Could you check a few things on this model? Use its own coordinates, in mm. Face numbers are marked on the shaded views. A direction names the side the tool comes from. Round coordinates to 2 decimals unless told otherwise and drop trailing zeros. Loops run counter-clockwise (first coordinate to the right, second up) from the corner with the lowest first, then second, coordinate; pieces in that order, holes last. Notation, with made-up numbers: M 34.25,-21 L 38.25,-21 A24 cw 38.25,2 Z; hole C -31.5,-25.5 d3. An arc over 180 degrees is marked long. Answer in a Markdown table with one row per item.
```python
from build123d import *

# Parameters (mm, degrees)
SKETCH018_R     = 1.75
PAD009_DEPTH    = 20
SKETCH019_W     = 27.500439
SKETCH019_H     = 11.45
SKETCH019_R     = 1.75
PAD010_DEPTH    = 4
SKETCH020_R     = 2.75
POCKET009_DEPTH = 8


with BuildPart() as part:
    # Sketch018 (on Face27 of Binder005) → Pad009 (new body)
    with BuildSketch(Plane.XZ.offset(-32.95)):
        Polygon((-0.000439, 13.05), (27.5, 13.05), (27.5, 1.6), (20.338297, 1.6), (20.338297, 3.6), (5.278297, 3.6), (5.278297, 1.6), (-0.000439, 1.6), align=None)
        with Locations((5.24978, 9.3)):
            Circle(SKETCH018_R, mode=Mode.SUBTRACT)
        with Locations((22.24978, 9.3)):
            Circle(SKETCH018_R, mode=Mode.SUBTRACT)
    extrude(amount=PAD009_DEPTH)

    # Sketch019 (on Face12 of Pad009) → Pad010 (join)
    with BuildSketch(Plane.XZ.offset(-12.95)):
        with Locations((13.74978, 7.325)):
            Rectangle(SKETCH019_W, SKETCH019_H)
        with Locations((5.24978, 9.3)):
            Circle(SKETCH019_R, mode=Mode.SUBTRACT)
        with Locations((22.24978, 9.3)):
            Circle(SKETCH019_R, mode=Mode.SUBTRACT)
    extrude(amount=PAD010_DEPTH)

    # Sketch020 (on Face1 of Pad010) → Pocket009 (cut)
    with BuildSketch(Plane.XZ.offset(-8.95)):
        with Locations((22.24978, 9.3)):
            Circle(SKETCH020_R)
        with Locations((5.24978, 9.3)):
            Circle(SKETCH020_R)
    extrude(amount=-POCKET009_DEPTH, mode=Mode.SUBTRACT)


solid = part.part
```
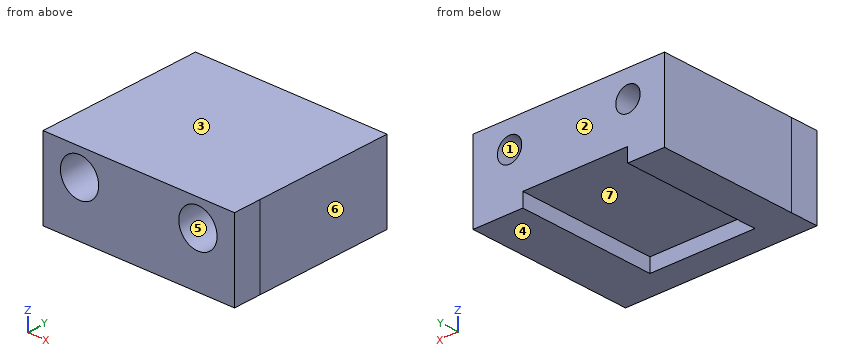
1) I want a section at C-C, the plane x = 19. Please give me the cut outline in (y, z), plus the area to 3 significant figures.
Computed:
| item | result |
|---|---|
| outline | M 8.95,1.6 L 12.95,1.6 L 12.95,3.6 L 32.95,3.6 L 32.95,13.05 L 8.95,13.05 Z |
| area | 235 mm² |
2) I want a section at B-B, the plane z = 9.3. Please give me the cut outline in (x, y).
Computed:
| item | result |
|---|---|
| outline | M 0,8.95 L 2.5,8.95 L 2.5,16.95 L 3.5,16.95 L 3.5,32.95 L 0,32.95 Z; M 7,16.95 L 8,16.95 L 8,8.95 L 19.5,8.95 L 19.5,16.95 L 20.5,16.95 L 20.5,32.95 L 7,32.95 Z; M 24,16.95 L 25,16.95 L 25,8.95 L 27.5,8.95 L 27.5,32.95 L 24,32.95 Z |
3) I want a section at D-D, the plane y = 11.5. Please give me the cut outline in (x, z).
Computed:
| item | result |
|---|---|
| outline | M 0,1.6 L 27.5,1.6 L 27.5,13.05 L 0,13.05 Z; hole C 5.25,9.3 d5.5; hole C 22.25,9.3 d5.5 |
4) I need wall thicknesses on line 1 (X direction, y = 27.75, z = 9.3); line 2 (X direction, y = 20.75, z = 8.25); line 3 (Z direction, x = 11.75, y = 20.5). Which ranges of each line are inside material? Lowest first, please.
Computed:
| item | result |
|---|---|
| line 1 | x = 0 to 3.5, 7 to 20.5, 24 to 27.5 |
| line 2 | x = 0 to 3.85, 6.65 to 20.85, 23.65 to 27.5 |
| line 3 | z = 3.6 to 13.05 |
5) Which directions (+Z, -Z, +X, -X, +Y, -Y) give clear straight access to the entire face, cutting with the end or side of a thin tool? Please do the marked faces 5, 6 and 7.
Computed:
| item | result |
|---|---|
| face 5 | -Y |
| face 6 | +Z, -Z, +X, +Y, -Y |
| face 7 | -Z, +Y |
6) I want a section at A-A, the plane y = 15. Please give me the cut outline in (x, z), plus the area to 3 significant figures.
Computed:
| item | result |
|---|---|
| outline | M 0,1.6 L 5.28,1.6 L 5.28,3.6 L 20.34,3.6 L 20.34,1.6 L 27.5,1.6 L 27.5,13.05 L 0,13.05 Z; hole C 5.25,9.3 d5.5; hole C 22.25,9.3 d5.5 |
| area | 237 mm² |
7) If we mould it in two halves opening along Z, with no side actions, what happens to the marked faces 1, 2, 3 and 4? For each: released by +Z, released by -Z, zero draft, split by the parting line, or undercut.
Computed:
| item | result |
|---|---|
| face 1 | undercut |
| face 2 | zero draft |
| face 3 | released by +Z |
| face 4 | released by -Z |
8) Will these pins go through, and if not, where does the flat tip stop? P1, Ø4.5, axis at x = 14.5, y = 26, coming from the -Z side; P2, Ø5.5, axis at x = 5.25, z = 9.3, coming from the +Y side; P3, Ø0.6, axis at x = 16.5, z = 3, coming from the +Y side.
Computed:
| item | result |
|---|---|
| P1 | stops at z = 3.6 |
| P2 | stops at y = 32.95 |
| P3 | stops at y = 12.95 |
